Check sheet for the drawn part. Datum: minimum x, y, z corner. Units: mm. A direction names the side the tool comes from. Give positions to 0.01 mm unless a question says otherwise; leave off trailing zeros. Order: outer loops, then holes, each group sorted by start corner. A loop starts at its lowest first (then second) coordinate and runs counter-clockwise, first axis right, second up. Notation, with made-up numbers: M 40.25,42.5 L 64.25,42.5 A24 ccw 64.25,71.5 Z; hole C -39,-40 d1. An arc over 180 degrees is marked long. Answer as CSV lines item,"result". Start each with the question number.
Q1. Go/stop test with flat-tipped pins: pin 1 (5 mm diameter, centred on x = 11.5, y = 65, fed in from +Z); pin 2 (1 mm diameter, centred on x = 19, y = 14.5, fed in from -Z); pin 3 (3 mm diameter, centred on x = 14, z = 15.5, fed in from +Y). Record where each tip stops, or that it passes through.
Q2. Section check D-D, the plane y = 48.5. Record the boundary of the cut face in (x, z).
Q3. Mould release check, pull along Z, two halves, no side actions. Record for the marked faces 1, 2 and 3: +Z half, -Z half, draft (parallel to the pull), parting line (faces both ways), or undercut.
Q4. Section check C-C, the plane z = 16. Record the boundary of the cut face in (x, y).
Q5. Set-up check for the marked faces 4, 5 and 6: record each of +Z, -Z, +X, -X, +Y, -Y from which the full face is reachable in a straight line by a thin tool's end or side.
Q6. Thickness scan on line 1 (Y direction, x = 18.75, z = 15); line 2 (Z direction, x = 20.5, y = 27); line 3 (Z direction, x = 22.25, y = 73.5) (1 decimal). Record the ranges inside material, lowest first.
Q7. Section check A-A, the plane y = 70.5. Record the boundary of the cut face in (x, z) (1 decimal), then the cut area to 3 significant figures.
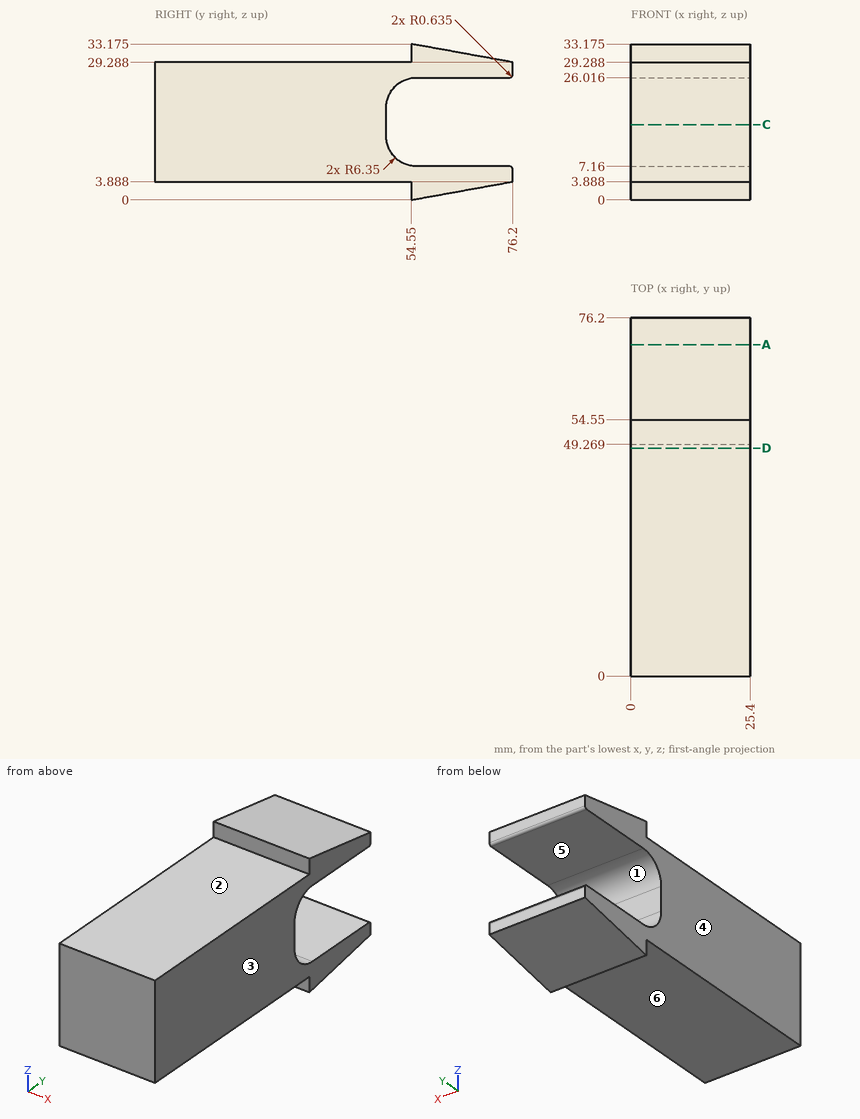
Answer block:
1,pin 1,"stops at z = 31.75"
1,pin 2,"stops at z = 3.89"
1,pin 3,"stops at y = 49.27"
2,outline,"M 0,3.89 L 25.4,3.89 L 25.4,29.29 L 0,29.29 Z"
3,face 1,"undercut"
3,face 2,"+Z half"
3,face 3,"draft"
4,outline,"M 0,0 L 25.4,0 L 25.4,49.27 L 0,49.27 Z"
5,face 4,"+Z, -Z, -X, +Y, -Y"
5,face 5,"+X, -X, +Y"
5,face 6,"-Z, +X, -X, -Y"
6,line 1,"y = 0 to 49.27"
6,line 2,"z = 3.89 to 29.29"
6,line 3,"z = 3.4 to 7.2, 26 to 29.8"
7,outline,"M 0,2.9 L 25.4,2.9 L 25.4,7.2 L 0,7.2 Z; M 0,26 L 25.4,26 L 25.4,30.3 L 0,30.3 Z"
7,area,"218 mm2"
